from build123d import *

# Parameters (mm, degrees)
FILLET1_R          = 2.54
SKETCH2_R          = 6.0325
CUT_EXTRUDE1_DEPTH = 2.54
FILLET2_R          = 2.54
SKETCH4_OUTSIDE_W  = 31.924
SKETCH4_OUTSIDE_H  = 31.924
SKETCH4_OUTSIDE_R  = 2.62
CUT_EXTRUDE2_DEPTH = 6.35


# Some blends are built 0.0001 mm under size
with BuildPart() as part:
    # Sketch1 → Base-Revolve (revolve)
    with BuildSketch(Plane.XY, mode=Mode.PRIVATE) as base_revolve_sk:
        with BuildLine():
            ThreePointArc((11.1125, 12.7), (6.622371939, 10.840128061), (4.7625, 6.35))
            Line((4.7625, 6.35), (3.175, 6.35))
            Line((3.175, 6.35), (3.175, 0))
            Line((3.175, 0), (0, 0))
            Line((0, 0), (0, 22.225))
            Line((0, 22.225), (11.1125, 22.225))
            Line((11.1125, 22.225), (11.1125, 12.7))
        make_face()
    revolve(base_revolve_sk.sketch.rotate(Axis((0, 0, 0), (0, 1, 0)), 90), axis=Axis((0, 0, 0), (0, 1, 0)))

    # Fillet1
    # the kernel refuses this fillet: 2.54 mm, written as the material it takes off along each edge
    with BuildSketch(Plane(origin=(0, 6.35, 0), x_dir=(0, 0, -1), z_dir=(1, 0, 0))) as fillet1_piece_1:
        with BuildLine():
            CenterArc((2.57175, 2.467324348), FILLET1_R, 283.739035174, 60.14756783)
            Line((3.175, 0), (3.187065, -0.049346487))
            ThreePointArc((3.187065, -0.049346487), (3.96875, -0.0508), (4.7625, -0.0508))
            Line((4.7625, -0.0508), (4.8133, 0))
            ThreePointArc((4.8133, 0), (4.875473976, 0.882851637), (5.060768571, 1.748275538))
            Line((5.060768571, 1.748275538), (5.011964286, 1.762374534))
        make_face()
    revolve(axis=Axis((0, 6.35, 0), (0, 1, 0)), mode=Mode.SUBTRACT)
    with BuildSketch(Plane(origin=(0, 22.225, 0), x_dir=(0, 0, -1), z_dir=(1, 0, 0))) as fillet1_piece_2:
        with BuildLine():
            CenterArc((11.1125 - FILLET1_R, -FILLET1_R), FILLET1_R, 0, 90)
            Line((11.1125, -FILLET1_R), (11.1125 + FILLET1_R * 0.02, -FILLET1_R))
            Line((11.1125 + FILLET1_R * 0.02, -FILLET1_R), (11.1125 + FILLET1_R * 0.02, FILLET1_R * 0.02))
            Line((11.1125 + FILLET1_R * 0.02, FILLET1_R * 0.02), (11.1125 - FILLET1_R, FILLET1_R * 0.02))
            Line((11.1125 - FILLET1_R, FILLET1_R * 0.02), (11.1125 - FILLET1_R, 0))
        make_face()
    revolve(axis=Axis((0, 22.225, 0), (0, 1, 0)), mode=Mode.SUBTRACT)
    with BuildSketch(Plane(origin=(0, 12.7, 0), x_dir=(0, 0, -1), z_dir=(1, 0, 0))) as fillet1_piece_3:
        with BuildLine():
            CenterArc((8.5725, 2.169418994), FILLET1_R, 286.601549599, 73.398450401)
            Line((11.1125, 2.169418994), (11.1633, 2.169418994))
            Line((11.1633, 2.169418994), (11.1633, 0))
            Line((11.1633, 0), (11.1125, -0.0508))
            ThreePointArc((11.1125, -0.0508), (10.203087128, -0.116791447), (9.312728571, -0.313383113))
            Line((9.312728571, -0.313383113), (9.298214286, -0.264700718))
        make_face()
    revolve(axis=Axis((0, 12.7, 0), (0, 1, 0)), mode=Mode.SUBTRACT)

    # Sketch2 → Cut-Extrude1 (cut)
    with BuildSketch(Plane(origin=(0, 22.225, 0), x_dir=(1, 0, 0), z_dir=(0, 1, 0))):
        with Locations(Location((0, 0, 0), (0, 0, 270))):
            Circle(SKETCH2_R)
    extrude(amount=-CUT_EXTRUDE1_DEPTH, mode=Mode.SUBTRACT)

    # Fillet2
    fillet2_edges = [part.edges().sort_by_distance(p)[0] for p in [
        (0, 19.685, -6.0325),
    ]]
    fillet(fillet2_edges, radius=FILLET2_R - 0.0001)  # a hair under: the kernel refuses the full size

    # Sketch4 outside → Cut-Extrude2 (cut)
    with BuildSketch(Plane.XZ):
        Rectangle(SKETCH4_OUTSIDE_W, SKETCH4_OUTSIDE_H)
        with Locations(Location((0, 0, 0), (0, 0, 270))):
            Circle(SKETCH4_OUTSIDE_R, mode=Mode.SUBTRACT)
    extrude(amount=-CUT_EXTRUDE2_DEPTH, mode=Mode.SUBTRACT)


solid = part.part
Read the model definition and answer for the solid it produces. Units are mm, in the model's axes. A direction names the side the tool comes from. Give positions to 0.01 mm unless a question says otherwise; leave off trailing zeros. Write each loop counter-clockwise with the first axis right and the second up, starting at its lowest first coordinate (ties: lowest second). Pieces come first, ordered by that corner, then holes. Notation, with made-up numbers: (71, 0) -> (101, 0) arc R34 cw to (101, 32) -> close; hole circle Ø6 at (72, -26). An arc over 180 degrees is marked (long way). Answer as a JSON object with one key per item and string values. Group by question number.
1) A tool of negligible diameter and unlimited length cuts with its end or side. For faces 4 (the flat face through (-6, 22.225, 2)), 5 (the cylindrical face through (2.598, 3.131, 0.341)), from which of +Z, -Z, +X, -X, +Y, -Y can it reach the whole face along a straight path? Write none if from no direction.
2) Find section C-C (y = 4.5). Write down the section's boundary in (x, z), and give its area (3 significant figures).
3) Consider L1, parallel to Y at x = 0, z = -0.75 (3 decimals); L2, parallel to Z at x = 5.25, y = 21; L3, parallel to Z at x = -4.25, y = 20.5. Determine where each line is inside the solid, lowest interval first. Write a range as from..to.
4) Find section D-D (y = 7). Write down the section's boundary in (x, z).
5) The mould has two halves that part along Z. Classify faces 1 (the flat face through (0, 6.35, 3)), 2 (the cylindrical face through (-7.5, 17.2, 8.2)), 3 (the flat face through (0, 19.685, 0)): +Z half, -Z half, draft (parallel to the pull), parting line (faces both ways), or undercut.
6) Each of these flat-tipped pins is pushed along its axis until it touches: P1, Ø5, axis at y = 9.5, z = -1, coming from the -X side; P2, Ø1.5, axis at x = 2.5, y = 2.5, coming from the -Z side; P3, Ø6, axis at y = 7.5, z = -5, coming from the -X side. Where does it stop, or does it pass through?
Values follow:
{
 "1": {"face 4": "+Z, -Z, +X, -X, +Y", "face 5": "-Y"},
 "2": {"outline": "circle Ø5.24 at (0, 0)", "area": "21.6 mm2"},
 "3": {"L1": "y = 0..19.685", "L2": "z = -9.38..-2.26, 2.26..9.38", "L3": "z = -10.12..-3.26, 3.26..10.12"},
 "4": {"outline": "circle Ø8.69 at (0, 0)"},
 "5": {"face 1": "draft", "face 2": "parting line", "face 3": "undercut"},
 "6": {"P1": "stops at x = -8.16", "P2": "stops at z = -1.95", "P3": "stops at x = -4.9"}
}
